from build123d import *

# Parameters (mm, degrees)
F0_R     = 67.31
F0_R_2   = 56.1246274
F1_DEPTH = 6.35
F0_R_3   = 49.7746274
F2_DEPTH = 19.05
F0_R_4   = 43.4246274
F0_R_5   = 37.0746274
F3_DEPTH = 25.4
F4_SIZE2 = 0.998358
F4_SIZE  = 19.04999
F5_SIZE2 = 19.04999
F5_SIZE  = 5.07999
F6_SIZE2 = 12.7
F6_SIZE  = 5.08
F7_DEPTH = 12.7
F9_DEPTH = 127
F10_R    = 1.27
F11_R    = 5.08


# Not quite as in the source:
# - a fillet or chamfer is up to 0.001 mm smaller than in the source, because OpenCascade refuses the exact size


with BuildPart() as f1:
    # F0 (on Top) → F1 (new body)
    with BuildSketch(Plane.XY):
        Circle(F0_R)
        Circle(F0_R_2, mode=Mode.SUBTRACT)
    extrude(amount=F1_DEPTH)



with BuildPart() as f2:
    # F0 (on Top) → F2 (new body)
    with BuildSketch(Plane.XY):
        Circle(F0_R_2)
        Circle(F0_R_3, mode=Mode.SUBTRACT)
    extrude(amount=-F2_DEPTH)


with BuildPart() as f1_1:
    add(f1.part)

    add(f2.part)  # F3 merges F2
    # F0 (on Top) → F3 (join)
    with BuildSketch(Plane.XY):
        Circle(F0_R_2)
        Circle(F0_R_3, mode=Mode.SUBTRACT)
        Circle(F0_R_3)
        Circle(F0_R_4, mode=Mode.SUBTRACT)
        Circle(F0_R_4)
        Circle(F0_R_5, mode=Mode.SUBTRACT)
    extrude(amount=F3_DEPTH)

    # F4 (size 19.05 and 0.9983681953 in the source; OpenCascade refuses exactly that, so slightly less here)
    f4_edges = [f1_1.edges().sort_by_distance(p)[0] for p in [
        (-56.124627, 0, -19.05),
    ]]
    f4_side = f1_1.faces().sort_by_distance((-56.124627, 0, -9.525))[0]
    chamfer(f4_edges, length=F4_SIZE, length2=F4_SIZE2, reference=f4_side)

    # F5 (size 5.08 and 19.05 in the source; OpenCascade refuses exactly that, so slightly less here)
    f5_edges = [f1_1.edges().sort_by_distance(p)[0] for p in [
        (-56.124627, 0, 25.4),
    ]]
    f5_side = f1_1.faces().sort_by_distance((-54.537183, 0, 25.4))[0]
    chamfer(f5_edges, length=F5_SIZE, length2=F5_SIZE2, reference=f5_side)

    # F6
    f6_edges = [f1_1.edges().sort_by_distance(p)[0] for p in [
        (-37.074627, 0, 25.4),
    ]]
    f6_side = f1_1.faces().sort_by_distance((-49.600877, 0, 25.4))[0]
    chamfer(f6_edges, length=F6_SIZE, length2=F6_SIZE2, reference=f6_side)

    # F0 (on Top) → F7 (join)
    with BuildSketch(Plane.XY):
        Circle(F0_R_5)
    extrude(amount=F7_DEPTH)

    # F8 (on face) → F9 (cut)
    with BuildSketch(Plane.XY.offset(25.4)):
        with BuildLine():
            ThreePointArc((-8.5611625958, -42.9912259739), (-10.7294880172, -43.2766914312), (-12.0608710658, -45.0117836011))
            Line((-12.0608710658, -45.0117836011), (-9.3007380172, -45.7513590225))
            Line((-9.3007380172, -45.7513590225), (-6.5406049686, -46.4909344439))
            ThreePointArc((-6.5406049686, -46.4909344439), (-6.4676843258, -46.1243376168), (-6.4432380172, -45.7513590225))
            ThreePointArc((-6.4432380172, -45.7513590225), (-7.0337308473, -44.0118232391), (-8.5611625958, -42.9912259739))
        make_face()
        with BuildLine():
            ThreePointArc((8.5611625958, -42.9912259739), (0, -43.8353626166), (-8.5611625958, -42.9912259739))
            Line((-8.5611625958, -42.9912259739), (-5.8010295472, -43.7308013952))
            Line((-5.8010295472, -43.7308013952), (-6.5406049686, -46.4909344439))
            Line((-6.5406049686, -46.4909344439), (-7.215923084, -49.0112559618))
            ThreePointArc((-7.215923084, -49.0112559618), (1.2593028677, -49.5235995582), (9.6975364764, -48.581174782))
            ThreePointArc((9.6975364764, -48.581174782), (6.5005137528, -46.3206132005), (8.5611625958, -42.9912259739))
        make_face()
        with BuildLine():
            Line((-9.3007380172, -45.7513590225), (-12.0608710658, -45.0117836011))
            ThreePointArc((-12.0608710658, -45.0117836011), (-11.7754056085, -47.1801090225), (-10.0403134386, -48.5114920711))
            ThreePointArc((-10.0403134386, -48.5114920711), (-9.8689864594, -48.5466359615), (-9.6975364764, -48.581174782))
            ThreePointArc((-9.6975364764, -48.581174782), (-7.7232039405, -48.1339400782), (-6.5406049686, -46.4909344439))
            Line((-6.5406049686, -46.4909344439), (-9.3007380172, -45.7513590225))
        make_face()
        with BuildLine():
            Line((-5.8010295472, -43.7308013952), (-8.5611625958, -42.9912259739))
            ThreePointArc((-8.5611625958, -42.9912259739), (-7.0337308473, -44.0118232391), (-6.4432380172, -45.7513590225))
            ThreePointArc((-6.4432380172, -45.7513590225), (-6.4676843258, -46.1243376168), (-6.5406049686, -46.4909344439))
            Line((-6.5406049686, -46.4909344439), (-5.8010295472, -43.7308013952))
        make_face()
        with BuildLine():
            ThreePointArc((-6.5406049686, -46.4909344439), (-7.7232039405, -48.1339400782), (-9.6975364764, -48.581174782))
            ThreePointArc((-9.6975364764, -48.581174782), (-8.4594634008, -48.8119886491), (-7.215923084, -49.0112559618))
            Line((-7.215923084, -49.0112559618), (-6.5406049686, -46.4909344439))
        make_face()
        with BuildLine():
            ThreePointArc((12.1582380172, -45.7513590225), (11.0402738006, -43.4843518526), (8.5611625958, -42.9912259739))
            ThreePointArc((8.5611625958, -42.9912259739), (6.5005137528, -46.3206132005), (9.6975364764, -48.581174782))
            ThreePointArc((9.6975364764, -48.581174782), (9.8689864594, -48.5466359615), (10.0403134386, -48.5114920711))
            ThreePointArc((10.0403134386, -48.5114920711), (11.5677451871, -47.4908948059), (12.1582380172, -45.7513590225))
        make_face()
    extrude(amount=-F9_DEPTH, mode=Mode.SUBTRACT)

    # F10
    f10_edges = [f1_1.edges().sort_by_distance(p)[0] for p in [
        (-67.31, 0, 6.35),
        (-51.044637, 0, 25.4),
        (-67.31, 0, 0),
        (-42.154627, 0, 25.4),
    ]]
    fillet(f10_edges, radius=F10_R)

    # F11
    f11_edges = [f1_1.edges().sort_by_distance(p)[0] for p in [
        (-37.074627, 0, 12.7),
    ]]
    fillet(f11_edges, radius=F11_R)


solid = f1_1.part
Geometry: final body of the model. Coordinates: model frame, mm. A direction names the side the tool comes from. Coordinates: 2 decimals unless noted, no trailing zeros. Order: outer loops, then holes, each group sorted by start corner. A loop starts at its lowest first (then second) coordinate and runs counter-clockwise, first axis right, second up.
(1) First-contact query: pin 1 (1 mm diameter, centred on y = 25, z = 5, fed in from -X); pin 2 (4 mm diameter, centred on x = -13.5, z = -8.5, fed in from +Y); pin 3 (4 mm diameter, centred on y = 39.5, z = 2, fed in from -X). Flat tips, straight axial feed; report the tip coordinate or a pass-through.
(2) Access query for faces 1 (the face through (0, 0, 12.7)), 2 (the face through (-1, 1, 0)), 3 (the face through (0.121, -43.835, 12.878)). Directions: +Z, -Z, +X, -X, +Y, -Y. A direction counts if a zero-diameter tool reaches every point of the face in a straight line with its end or side. Return the directions, or none.
(3) Section query B-B (z = -10.5). Return the cut outline in (x, y).
(4) Material intervals for probe 1 along Y at (x, z) = (0, -5.75); probe 2 along Y at (x, z) = (0, -11); probe 3 along Z at (x, y) = (7, -26), sorted ascending.
(5) Draft query along X for faces 4 (the face through (-10.79, -48.59, -9.39)), 5 (the face through (-14.59, -65.71, 3.15)), 6 (the face through (-8.4, 49.3, -19.05)). Return one class per face: pulls with the +X half, pulls with the -X half, needs draft (parallel to the pull), parting line crosses it, or undercut.
Solution:
1. pin 1: stops at x = -62.69
1. pin 2: stops at y = 54.49
1. pin 3: stops at x = -55.9
2. face 1: +Z
2. face 2: -Z
2. face 3: +Z, -Z
3. outline: circle Ø111.15 at (0, 0); hole circle Ø99.55 at (0, 0)
4. probe 1: y = -55.82 to -49.77, 49.77 to 55.82
4. probe 2: y = -55.55 to -49.77, 49.77 to 55.55
4. probe 3: z = 0 to 12.7
5. face 4: undercut
5. face 5: parting line crosses it
5. face 6: needs draft
